Autodesk Inventor part; units mm, degrees
ref_plane "YZ Plane" through (0, 0, 0) normal (1, 0, 0) x (0, 1, 0)
ref_plane "XZ Plane" through (0, 0, 0) normal (0, 1, 0) x (-1, 0, 0)
ref_plane "XY Plane" through (0, 0, 0) normal (0, 0, 1) x (1, 0, 0)
sketch "Sketch1" plane through (0, 0, 0) normal (0, 1, 0) x (-1, 0, 0)
  line L0 (-15.65, -21.15) -> (15.65, -21.15)
  line L1 (21.15, -15.65) -> (21.15, 15.65)
  line L2 (15.65, 21.15) -> (-15.65, 21.15)
  line L3 (-21.15, 15.65) -> (-21.15, -15.65)
  line L4 (-21.15, -21.15) -> (21.15, 21.15) construction
  line L5 (21.15, -21.15) -> (-21.15, 21.15) construction
  line L6 (15.65, 21.15) -> (21.15, 15.65)
  line L7 (-15.65, 21.15) -> (-21.15, 15.65)
  line L8 (-21.15, -15.65) -> (-15.65, -21.15)
  line L9 (15.65, -21.15) -> (21.15, -15.65)
  point P0 (0, 0)
  dimension "d0" = 42.3
  dimension "d1" = 42.3
  dimension "d2" = 5.5
  dimension "d3" = 5.5
  dimension "d4" = 5.5
  dimension "d5" = 5.5
  dimension "d6" = 5.5
  dimension "d7" = 5.5
  dimension "d8" = 5.5
  dimension "d9" = 5.5
extrude "Extrusion1" add sketch "Sketch1" along normal blind 47
sketch "Sketch2" plane through (0, 47, 0) normal (0, 1, 0) x (1, 0, 0)
  circle A0 centre (0, 0) radius 11
  dimension "d12" = 22
extrude "Extrusion2" add sketch "Sketch2" along normal blind 2
sketch "Sketch3" plane through (0, 49, 0) normal (0, 1, 0) x (1, 0, 0)
  circle A0 centre (0, 0) radius 2.5
  dimension "d15" = 5
extrude "Extrusion3" add sketch "Sketch3" along normal blind 22
sketch "Sketch4" plane through (0, 47, 0) normal (0, 1, 0) x (1, 0, 0)
  line L0 (89.125, 0) -> (-55.025, 0)
  line L1 (0, 94.2917) -> (0, -108.2417)
  point P0 (0, 0)
  point P1 (15.5, 15.5)
  point P2 (15.5, -15.5)
  point P3 (-15.5, 15.5)
  point P4 (-15.5, -15.5)
  dimension "d18" = 31
  dimension "d19" = 31
hole "Hole1" at (15.5, 47, -15.5) at (15.5, 47, 15.5) at (-15.5, 47, -15.5) at (-15.5, 47, 15.5) direction (0, -1, 0) diameter 2.4638 depth 5 tip angle 118
sketch "Sketch6" plane through (15.65, 0, -21.15) normal (0, 0, -1) x (-1, 0, 0)
  line L0 (15.65, -0.9377) -> (15.65, 31.0797)
  line L1 (31.3, 0) -> (0, 0)
  circle A0 centre (11.84, 2.54) radius 0.8268
  circle A1 centre (14.38, 2.54) radius 0.8268
  line L2 (6.0146, 2.54) -> (34.3637, 2.54)
  circle A2 centre (19.46, 2.54) radius 0.8268
  circle A3 centre (16.92, 2.54) radius 0.8268
  point P0 (15.65, 0)
  point P1 (15.65, 0)
  dimension "d31" = 2.54
  dimension "d32" = 2.54
  dimension "d33" = 1.6536
  dimension "d34" = 1.6536
  dimension "d36" = 2.54
extrude "Extrusion6" add sketch "Sketch6" along normal blind 5.08
equation "\"d1\" = d0"
equation "\"d3\" = d2"
equation "\"d4\" = d2"
equation "\"d5\" = d4"
equation "\"d6\" = d2"
equation "\"d7\" = d6"
equation "\"d8\" = d2"
equation "\"d9\" = d8"
equation "\"d32\" = d31"
equation "\"d34\" = d33"
properties part number "Stepper_Motor"
Design review of the part built by this model. Coordinates are the model's own, in mm. A direction names the side the tool comes from. Coordinates: 2 decimals unless noted, no trailing zeros. Order: outer loops, then holes, each group sorted by start corner. A loop starts at its lowest first (then second) coordinate and runs counter-clockwise, first axis right, second up.
1) For faces 1 (the cylindrical face through (-2.06, 2.29, -23.65)), 2 (the cylindrical face through (14.46, 44.46, 16.16)), 3 (the flat face through (-21.15, 23, 0)), list the 3-axis set-ups (+Z, -Z, +X, -X, +Y, -Y) from which the entire face can be reached by the end or side of a thin tool; tool diameter is ignored.
2) Mouldability with a two-part tool opening along X and no side actions: class faces 4 (the flat face through (18.4, 23.2, 18.4)), 5 (the cylindrical face through (-0.54, 59.85, -2.44)), 6 (the flat face through (10, 47, -9)), 7 (the conical face through (-15.288, 41.388, 15.472)) as +X half, -X half, draft (parallel to the pull), parting line (faces both ways), or undercut.
3) Take a section at B-B, the plane y = 24.5. Give the boundary of the cut face in (x, z).
4) Take a section at D-D, the plane x = 3.81. Give the boundary of the cut face in (y, z), and give its area (3 significant figures).
5) Wall thickness on line 1 along Z through (x, y) = (-15.5, 45.25); line 2 along X through (y, z) = (44, 15): over which ranges is each line inside the solid? List them lowest first.
6) Clearance check with flat-ended pins moving along their axes: pin 1 (4 mm diameter, centred on x = -15.5, z = 15.5, fed in from +Y); pin 2 (9.5 mm diameter, centred on x = 4, y = 29.5, fed in from -Z); pin 3 (1.5 mm diameter, centred on x = -15.5, z = -15.5, fed in from -Y); pin 4 (1.5 mm diameter, centred on y = 44, z = -20.5, fed in from +X). State where each tip first meets the part, or that it passes through.
7) Take a section at C-C, the plane x = -10. Give the boundary of the cut face in (y, z).
8) Take a section at A-A, the plane z = 0. Give the boundary of the cut face in (x, y), and give its area (3 significant figures).
Returned:
1. face 1: -Z
1. face 2: +Y
1. face 3: +Z, -Z, -X, +Y, -Y
2. face 4: +X half
2. face 5: parting line
2. face 6: draft
2. face 7: undercut
3. outline: (-21.15, -15.65) - (-15.65, -21.15) - (15.65, -21.15) - (21.15, -15.65) - (21.15, 15.65) - (15.65, 21.15) - (-15.65, 21.15) - (-21.15, 15.65) - close
4. outline: (0, -21.15) - (1.71, -21.15) - (1.71, -26.23) - (3.37, -26.23) - (3.37, -21.15) - (47, -21.15) - (47, -10.32) - (49, -10.32) - (49, 10.32) - (47, 10.32) - (47, 21.15) - (0, 21.15) - close
4. area: 2,040 mm2
5. line 1: z = -21.15 to -16.73, -14.27 to 14.27, 16.73 to 21.15
5. line 2: x = -21.15 to -16.63, -14.37 to 14.37, 16.63 to 21.15
6. pin 1: stops at y = 47
6. pin 2: stops at z = -21.15
6. pin 3: stops at y = 0
6. pin 4: stops at x = 17.05
7. outline: (0, -21.15) - (47, -21.15) - (47, -4.58) - (49, -4.58) - (49, 4.58) - (47, 4.58) - (47, 21.15) - (0, 21.15) - close
8. outline: (-21.15, 0) - (21.15, 0) - (21.15, 47) - (11, 47) - (11, 49) - (2.5, 49) - (2.5, 71) - (-2.5, 71) - (-2.5, 49) - (-11, 49) - (-11, 47) - (-21.15, 47) - close
8. area: 2,140 mm2
